Design review of the part built by this model. Coordinates are the model's own, in mm. Face numbers are marked on the shaded views. A direction names the side the tool comes from. Give positions to 0.01 mm unless a question says otherwise; leave off trailing zeros. Order: outer loops, then holes, each group sorted by start corner. A loop starts at its lowest first (then second) coordinate and runs counter-clockwise, first axis right, second up. Notation, with made-up numbers: (36.25, 40) -> (88.25, 40) arc R11 cw to (88.25, 57) -> close; hole circle Ø9 at (-22, -13.75). An arc over 180 degrees is marked (long way). Use a Markdown table: item, result. Add a question column.
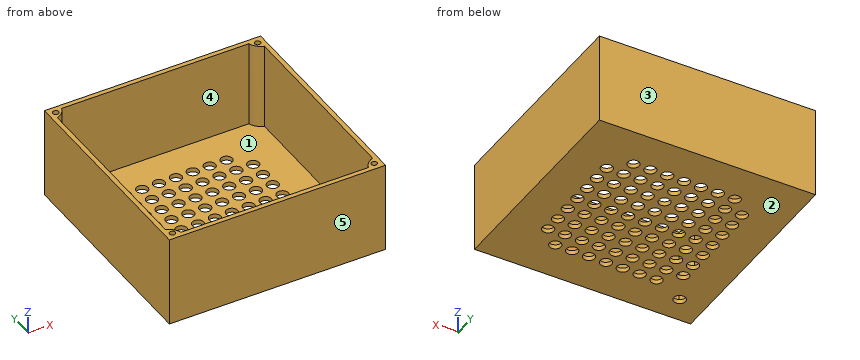
```python
from build123d import *

# Parameters (mm, degrees)
SKETCH_W     = 150
SKETCH_H     = 150
SKETCH_R     = 4
SKETCH_R_2   = 4.1
PAD_DEPTH    = 3
SKETCH001_W  = 150
SKETCH001_H  = 150
PAD001_DEPTH = 60
SKETCH002_R  = 2
POCKET_DEPTH = 10


with BuildPart() as part:
    # Sketch → Pad (new body)
    with BuildSketch(Plane.XY):
        Rectangle(SKETCH_W, SKETCH_H)
        with Locations((-35.17664, 46.860641)):
            Circle(SKETCH_R, mode=Mode.SUBTRACT)
        with Locations((-23.457463, 46.865997)):
            Circle(SKETCH_R, mode=Mode.SUBTRACT)
        with Locations((-11.738286, 46.871353)):
            Circle(SKETCH_R, mode=Mode.SUBTRACT)
        with Locations((-0.019109, 46.876709)):
            Circle(SKETCH_R, mode=Mode.SUBTRACT)
        with Locations((11.700068, 46.882065)):
            Circle(SKETCH_R, mode=Mode.SUBTRACT)
        with Locations((23.419245, 46.887421)):
            Circle(SKETCH_R, mode=Mode.SUBTRACT)
        with Locations((35.138422, 46.892777)):
            Circle(SKETCH_R, mode=Mode.SUBTRACT)
        with Locations((-46.892776, 35.136107)):
            Circle(SKETCH_R, mode=Mode.SUBTRACT)
        with Locations((-35.173599, 35.141463)):
            Circle(SKETCH_R, mode=Mode.SUBTRACT)
        with Locations((-23.454422, 35.146819)):
            Circle(SKETCH_R, mode=Mode.SUBTRACT)
        with Locations((-11.735245, 35.152175)):
            Circle(SKETCH_R, mode=Mode.SUBTRACT)
        with Locations((-0.016068, 35.157531)):
            Circle(SKETCH_R, mode=Mode.SUBTRACT)
        with Locations((11.703109, 35.162887)):
            Circle(SKETCH_R, mode=Mode.SUBTRACT)
        with Locations((23.422286, 35.168243)):
            Circle(SKETCH_R, mode=Mode.SUBTRACT)
        with Locations((35.141463, 35.173599)):
            Circle(SKETCH_R, mode=Mode.SUBTRACT)
        with Locations((46.86064, 35.178955)):
            Circle(SKETCH_R, mode=Mode.SUBTRACT)
        with Locations((-46.88742, 23.41693)):
            Circle(SKETCH_R, mode=Mode.SUBTRACT)
        with Locations((-35.168243, 23.422286)):
            Circle(SKETCH_R, mode=Mode.SUBTRACT)
        with Locations((-23.449066, 23.427642)):
            Circle(SKETCH_R, mode=Mode.SUBTRACT)
        with Locations((-11.729889, 23.432998)):
            Circle(SKETCH_R, mode=Mode.SUBTRACT)
        with Locations((-0.010712, 23.438354)):
            Circle(SKETCH_R, mode=Mode.SUBTRACT)
        with Locations((11.708465, 23.44371)):
            Circle(SKETCH_R, mode=Mode.SUBTRACT)
        with Locations((23.427642, 23.449066)):
            Circle(SKETCH_R, mode=Mode.SUBTRACT)
        with Locations((35.146819, 23.454422)):
            Circle(SKETCH_R, mode=Mode.SUBTRACT)
        with Locations((46.865996, 23.459778)):
            Circle(SKETCH_R, mode=Mode.SUBTRACT)
        with Locations((-46.882064, 11.697753)):
            Circle(SKETCH_R, mode=Mode.SUBTRACT)
        with Locations((-35.162887, 11.703109)):
            Circle(SKETCH_R, mode=Mode.SUBTRACT)
        with Locations((-23.44371, 11.708465)):
            Circle(SKETCH_R, mode=Mode.SUBTRACT)
        with Locations((-11.724533, 11.713821)):
            Circle(SKETCH_R, mode=Mode.SUBTRACT)
        with Locations((-0.005356, 11.719177)):
            Circle(SKETCH_R, mode=Mode.SUBTRACT)
        with Locations((11.713821, 11.724533)):
            Circle(SKETCH_R, mode=Mode.SUBTRACT)
        with Locations((23.432998, 11.729889)):
            Circle(SKETCH_R, mode=Mode.SUBTRACT)
        with Locations((35.152175, 11.735245)):
            Circle(SKETCH_R, mode=Mode.SUBTRACT)
        with Locations((46.871352, 11.740601)):
            Circle(SKETCH_R, mode=Mode.SUBTRACT)
        with Locations((-46.876708, -0.021424)):
            Circle(SKETCH_R, mode=Mode.SUBTRACT)
        with Locations((-35.157531, -0.016068)):
            Circle(SKETCH_R, mode=Mode.SUBTRACT)
        with Locations((-23.438354, -0.010712)):
            Circle(SKETCH_R, mode=Mode.SUBTRACT)
        with Locations((-11.719177, -0.005356)):
            Circle(SKETCH_R, mode=Mode.SUBTRACT)
        Circle(SKETCH_R, mode=Mode.SUBTRACT)
        with Locations((11.719177, 0.005356)):
            Circle(SKETCH_R, mode=Mode.SUBTRACT)
        with Locations((23.438354, 0.010712)):
            Circle(SKETCH_R, mode=Mode.SUBTRACT)
        with Locations((35.157531, 0.016068)):
            Circle(SKETCH_R, mode=Mode.SUBTRACT)
        with Locations((46.876708, 0.021424)):
            Circle(SKETCH_R, mode=Mode.SUBTRACT)
        with Locations((-46.871352, -11.740601)):
            Circle(SKETCH_R, mode=Mode.SUBTRACT)
        with Locations((-35.152175, -11.735245)):
            Circle(SKETCH_R, mode=Mode.SUBTRACT)
        with Locations((-23.432998, -11.729889)):
            Circle(SKETCH_R, mode=Mode.SUBTRACT)
        with Locations((-11.713821, -11.724533)):
            Circle(SKETCH_R, mode=Mode.SUBTRACT)
        with Locations((0.005356, -11.719177)):
            Circle(SKETCH_R, mode=Mode.SUBTRACT)
        with Locations((11.724533, -11.713821)):
            Circle(SKETCH_R, mode=Mode.SUBTRACT)
        with Locations((23.44371, -11.708465)):
            Circle(SKETCH_R, mode=Mode.SUBTRACT)
        with Locations((35.162887, -11.703109)):
            Circle(SKETCH_R, mode=Mode.SUBTRACT)
        with Locations((46.882064, -11.697753)):
            Circle(SKETCH_R, mode=Mode.SUBTRACT)
        with Locations((-46.865996, -23.459778)):
            Circle(SKETCH_R, mode=Mode.SUBTRACT)
        with Locations((-35.146819, -23.454422)):
            Circle(SKETCH_R, mode=Mode.SUBTRACT)
        with Locations((-23.427642, -23.449066)):
            Circle(SKETCH_R, mode=Mode.SUBTRACT)
        with Locations((-11.708465, -23.44371)):
            Circle(SKETCH_R, mode=Mode.SUBTRACT)
        with Locations((0.010712, -23.438354)):
            Circle(SKETCH_R, mode=Mode.SUBTRACT)
        with Locations((11.729889, -23.432998)):
            Circle(SKETCH_R, mode=Mode.SUBTRACT)
        with Locations((23.449066, -23.427642)):
            Circle(SKETCH_R, mode=Mode.SUBTRACT)
        with Locations((35.168243, -23.422286)):
            Circle(SKETCH_R, mode=Mode.SUBTRACT)
        with Locations((46.88742, -23.41693)):
            Circle(SKETCH_R, mode=Mode.SUBTRACT)
        with Locations((-46.86064, -35.178955)):
            Circle(SKETCH_R, mode=Mode.SUBTRACT)
        with Locations((-35.141463, -35.173599)):
            Circle(SKETCH_R, mode=Mode.SUBTRACT)
        with Locations((-23.422286, -35.168243)):
            Circle(SKETCH_R, mode=Mode.SUBTRACT)
        with Locations((-11.703109, -35.162887)):
            Circle(SKETCH_R, mode=Mode.SUBTRACT)
        with Locations((0.016068, -35.157531)):
            Circle(SKETCH_R, mode=Mode.SUBTRACT)
        with Locations((11.735245, -35.152175)):
            Circle(SKETCH_R, mode=Mode.SUBTRACT)
        with Locations((23.454422, -35.146819)):
            Circle(SKETCH_R, mode=Mode.SUBTRACT)
        with Locations((35.173599, -35.141463)):
            Circle(SKETCH_R, mode=Mode.SUBTRACT)
        with Locations((46.892776, -35.136107)):
            Circle(SKETCH_R, mode=Mode.SUBTRACT)
        with Locations((-35.136049, -46.892776)):
            Circle(SKETCH_R, mode=Mode.SUBTRACT)
        with Locations((-23.416872, -46.88742)):
            Circle(SKETCH_R, mode=Mode.SUBTRACT)
        with Locations((-11.697695, -46.882064)):
            Circle(SKETCH_R, mode=Mode.SUBTRACT)
        with Locations((0.021482, -46.876708)):
            Circle(SKETCH_R, mode=Mode.SUBTRACT)
        with Locations((11.740659, -46.871352)):
            Circle(SKETCH_R, mode=Mode.SUBTRACT)
        with Locations((23.459836, -46.865996)):
            Circle(SKETCH_R, mode=Mode.SUBTRACT)
        with Locations((35.179013, -46.86064)):
            Circle(SKETCH_R, mode=Mode.SUBTRACT)
        with Locations((-57, -57)):
            Circle(SKETCH_R_2, mode=Mode.SUBTRACT)
    extrude(amount=PAD_DEPTH)

    # Sketch001 (on DatumPlane) → Pad001 (join)
    with BuildSketch(Plane.XY.offset(3)):
        Rectangle(SKETCH001_W, SKETCH001_H)
        with BuildLine():
            Line((-65, 71.825478), (65, 71.825478))
            ThreePointArc((65, 71.825478), (67.581186, 67.581186), (71.825478, 65))
            Line((71.825478, 65), (71.825478, -65))
            ThreePointArc((71.825478, -65), (67.581186, -67.581186), (65, -71.825478))
            Line((65, -71.825478), (-65, -71.825478))
            ThreePointArc((-65, -71.825478), (-67.581186, -67.581186), (-71.825478, -65))
            Line((-71.825478, -65), (-71.825478, 65))
            ThreePointArc((-71.825478, 65), (-67.581186, 67.581186), (-65, 71.825478))
        make_face(mode=Mode.SUBTRACT)
    extrude(amount=PAD001_DEPTH)

    # Sketch002 (on DatumPlane) → Pocket (cut)
    with BuildSketch(Plane.XY.offset(63)):
        with Locations((-70, 70)):
            Circle(SKETCH002_R)
        with Locations((70, 70)):
            Circle(SKETCH002_R)
        with Locations((-70, -70)):
            Circle(SKETCH002_R)
        with Locations((70, -70)):
            Circle(SKETCH002_R)
    extrude(amount=-POCKET_DEPTH, mode=Mode.SUBTRACT)


solid = part.part
```
1) Add section A-A (x = -57). Give the boundary of the cut face in (y, z), then the cut area to 3 significant figures.
2) For L1, parallel to X at y = -29, z = 38; L2, parallel to Y at x = -70, z = 60, list the stretches that pass through material, from the lowest coordinate up. Write a range as [from, to].
3) The part is to be moulded in two halves that separate along Y. For the marked faces 1, 2 and 3, say which applies: +Y half, -Y half, draft (parallel to the pull), parting line (faces both ways), or undercut.
4) Insertion check: pin 1 (13 mm diameter, centred on x = -23.45, y = 35.15, fed in from -Z); pin 2 (9 mm diameter, centred on x = -46.87, y = -23.46, fed in from +Z). Each pin has a flat end and moves straight along its axis. Give the tip position at first contact, or say it passes through.
5) Add section D-D (x = 46.5). Give the number of separate pieces and of enclosed holes in the cut face, then the cut area to 3 significant figures.
6) Machinability: for the marked faces 4 and 5, which of the approach directions +Z, -Z, +X, -X, +Y, -Y give a long, thin tool a straight path to every point of the face, cutting with its end or side? Answer none if there is none.
7) Add section B-B (z = 31.5). Give the boundary of the cut face in (x, y).
Worked answers:
| question | item | result |
|---|---|---|
| 1 | outline | (-75, 0) -> (-61.1, 0) -> (-61.1, 3) -> (-71.83, 3) -> (-71.83, 63) -> (-75, 63) -> close; (-52.9, 0) -> (75, 0) -> (75, 63) -> (71.83, 63) -> (71.83, 3) -> (-52.9, 3) -> close |
| 1 | area | 806 mm^2 |
| 2 | L1 | [-75, -71.83], [71.83, 75] |
| 2 | L2 | [-75, -72], [-68, -65.78], [65.78, 68], [72, 75] |
| 3 | face 1 | undercut |
| 3 | face 2 | draft |
| 3 | face 3 | +Y half |
| 4 | pin 1 | z = 0 |
| 4 | pin 2 | z = 3 |
| 5 | separate pieces | 8 |
| 5 | enclosed holes | 0 |
| 5 | area | 664 mm^2 |
| 6 | face 4 | +Z |
| 6 | face 5 | +Z, -Z, +X, -X, -Y |
| 7 | outline | (-75, -75) -> (75, -75) -> (75, 75) -> (-75, 75) -> close; hole (-71.83, -65) arc R10.49 cw to (-65, -71.83) -> (65, -71.83) arc R10.49 cw to (71.83, -65) -> (71.83, 65) arc R10.49 cw to (65, 71.83) -> (-65, 71.83) arc R10.49 cw to (-71.83, 65) -> close |
